The listing builds one solid part. Answer for the finished solid, in the listing's coordinates (mm). A direction names the side the tool comes from. Round coordinates to 2 decimals unless told otherwise and drop trailing zeros. Loops run counter-clockwise (first coordinate to the right, second up) from the corner with the lowest first, then second, coordinate; pieces in that order, holes last. Notation, with made-up numbers: (14, 44) - (54, 44) arc R13 cw to (54, 65) - close; hole circle Ø6 at (-3.75, 26). An arc over 180 degrees is marked (long way). One line per question, with ' | ' between items. Start each with the question number.
from build123d import *

# Parameters (mm, degrees)
IZIM1_W                     = 73
IZIM1_H                     = 52
Y_KSEKLIK_EKSTR_ZYON1_DEPTH = 56
IZIM2_W                     = 37
IZIM2_H                     = 30
KES_EKSTR_ZYON1_DEPTH       = 106.683489723
RADYUS1_R                   = 26
RADYUS2_R                   = 26
RADYUS3_R                   = 26
RADYUS5_R                   = 26


with BuildPart() as part:
    # Çizim1 → Yükseklik-Ekstrüzyon1 (new body)
    with BuildSketch(Plane.XY):
        with Locations((36.5, 26)):
            Rectangle(IZIM1_W, IZIM1_H)
    extrude(amount=Y_KSEKLIK_EKSTR_ZYON1_DEPTH)

    # Çizim2 → Kes-Ekstrüzyon1 (cut, through all)
    with BuildSketch(Plane(origin=(0, 52, 0), x_dir=(1, 0, 0), z_dir=(0, 1, 0))):
        with Locations((54.5, -28)):
            Rectangle(IZIM2_W, IZIM2_H)
    extrude(amount=-KES_EKSTR_ZYON1_DEPTH, mode=Mode.SUBTRACT)

    # Radyus1
    radyus1_edges = [part.edges().sort_by_distance(p)[0] for p in [
        (73, 52, 49.5),
    ]]
    fillet(radyus1_edges, radius=RADYUS1_R)

    # Radyus2
    radyus2_edges = [part.edges().sort_by_distance(p)[0] for p in [
        (73, 0, 49.5),
    ]]
    fillet(radyus2_edges, radius=RADYUS2_R - 0.0001)  # a hair under: the kernel refuses the full size

    # Radyus3
    radyus3_edges = [part.edges().sort_by_distance(p)[0] for p in [
        (73, 52, 6.5),
    ]]
    fillet(radyus3_edges, radius=RADYUS3_R)

    # Radyus5
    radyus5_edges = [part.edges().sort_by_distance(p)[0] for p in [
        (73, 0, 6.5),
    ]]
    fillet(radyus5_edges, radius=RADYUS5_R - 0.0001)  # a hair under: the kernel refuses the full size


solid = part.part
(1) A tool of negligible diameter and unlimited length cuts with its end or side. For faces 1 (the flat face through (36, 26, 28)), 2 (the cylindrical face through (65.18, 44.59, 6.59)), from which of +Z, -Z, +X, -X, +Y, -Y can it reach the whole face along a straight path? Write none if from no direction.
(2) Consider L1, parallel to Z at x = 51, y = 16.5; L2, parallel to X at y = 25.5, z = 22.5; L3, parallel to X at y = 15.5, z = 45. Determine where each line is inside the solid, lowest interval first.
(3) Each of these flat-tipped pins is pushed along its axis until it touches: P1, Ø8, axis at y = 11.5, z = 21.5, coming from the -X side; P2, Ø1.5, axis at y = 5.5, z = 32, coming from the +X side. Where does it stop, or does it pass through?
(4) Find section D-D on x = 61. Write down the section's boundary in (y, z).
(5) Find section B-B on y = 48. Write down the section's boundary in (x, z), plus the area to 3 significant figures.
(6) Determine the mould class of faces 3 (the cylindrical face through (65.18, 44.59, 49.59)), 4 (the flat face through (36, 26, 0)), 5 (the flat face through (50, 26, 13)) for opening direction Z: pulls with the +Z half, pulls with the -Z half, needs draft (parallel to the pull), parting line crosses it, or undercut.
(7) Find section A-A on x = 46. Write down the section's boundary in (y, z).
Answer below:
1) face 1: +X, +Y, -Y | face 2: +Z, -Z, +X, +Y
2) L1: 0 to 13, 43 to 56 | L2: 0 to 36 | L3: 0 to 70.79
3) P1: x = 0 | P2: x = 36
4) outline: (4.09, 0) - (47.91, 0) - (47.91, 13) - (4.09, 13) - close; (4.09, 43) - (47.91, 43) - (47.91, 56) - (4.09, 56) - close
5) outline: (0, 0) - (60.86, 0) - (60.86, 13) - (36, 13) - (36, 43) - (60.86, 43) - (60.86, 56) - (0, 56) - close | area: 2,660 mm2
6) face 3: needs draft | face 4: pulls with the -Z half | face 5: undercut
7) outline: (0, 0) - (52, 0) - (52, 13) - (0, 13) - close; (0, 43) - (52, 43) - (52, 56) - (0, 56) - close
